Autodesk Inventor part; units mm, degrees
ref_plane "YZ Plane" through (0, 0, 0) normal (1, 0, 0) x (0, 1, 0)
ref_plane "XZ Plane" through (0, 0, 0) normal (0, 1, 0) x (-1, 0, 0)
ref_plane "XY Plane" through (0, 0, 0) normal (0, 0, 1) x (1, 0, 0)
sketch "Sketch1" plane through (0, 0, 0) normal (0, 1, 0) x (-1, 0, 0)
  circle A0 centre (0, 0) radius 9.525
  dimension "d0" = 19.05
extrude "Extrusion1" add sketch "Sketch1" along normal mid plane 30.48
sketch "Sketch3" plane through (0, 15.24, 0) normal (0, 1, 0) x (1, 0, 0)
  point P0 (0, 0)
  point P1 (0, 0)
hole "Hole1" at (0, 15.24, 0) direction (0, -1, 0) diameter 7.9375 end through all
sketch "Sketch4" plane through (0, 15.24, 0) normal (0, 1, 0) x (1, 0, 0)
  point P0 (0, 0)
  point P1 (0, 0)
hole "Hole2" at (0, 15.24, 0) direction (0, -1, 0) diameter 12.3031 depth 10.16 tip angle 118
sketch "Sketch5" plane through (0, 15.24, 0) normal (0, 1, 0) x (1, 0, 0)
  circle A0 centre (0, 0) radius 6.3627
  dimension "d20" = 12.7254
extrude "Extrusion3" cut sketch "Sketch5" against normal blind 11.43
sketch "Sketch6" plane through (0, 15.24, 0) normal (0, 1, 0) x (1, 0, 0)
  circle A0 centre (0, 0) radius 6.477
  dimension "d23" = 12.954
extrude "Extrusion4" cut sketch "Sketch6" against normal blind 2.54
sketch "Sketch7" plane through (0, -15.24, 0) normal (0, -1, 0) x (1, 0, 0)
  circle A0 centre (0, 0) radius 9.525
  circle A1 centre (0, 0) radius 9.525
  circle A2 centre (0, 0) radius 5.5753
  dimension "d26" = 11.1506
extrude "Extrusion5" cut sketch "Sketch7" against normal blind 15.24
sketch "Sketch9" plane through (0, 0, 0) normal (0, 0, 1) x (1, 0, 0)
  line L0 (3.9688, -15.24) -> (-3.9688, -15.24)
  line L1 (0, -15.24) -> (0, -4.064) construction
  line L2 (0, -15.24) -> (11.176, -15.24) construction
  line L3 (0, -4.064) -> (5.5753, -4.064) construction
  line L4 (5.5753, -15.24) -> (5.5753, 0)
  line L5 (5.7023, -2.794) -> (5.4483, -2.794)
  line L6 (5.4483, -2.794) -> (5.4483, -5.334)
  line L7 (5.4483, -5.334) -> (5.7023, -5.334)
  line L8 (5.7023, -5.334) -> (5.7023, -2.794)
  line L9 (5.7023, -2.794) -> (5.4483, -5.334) construction
  line L10 (5.4483, -2.794) -> (5.7023, -5.334) construction
  point P0 (0, 0)
  dimension "d35" = 11.176
  dimension "d36" = 90
  dimension "d38" = 90
  dimension "d39" = 0.254
  dimension "d40" = 2.54
revolve "Revolution1" cut sketch "Sketch9" angle 360 about axis through (0, -15.24, 0) along (0, 1, 0)
chamfer "Chamfer2" distance 1.5875 angle 45 1 edges at (9.525, 0, 0)
properties part number "fridge bushing" material "Brass"
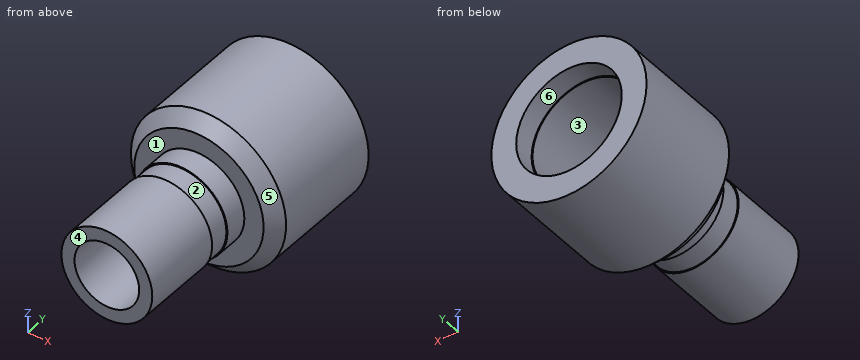
Geometry: final body of the model. Coordinates: model frame, mm. Face numbers are marked on the shaded views. A direction names the side the tool comes from. Coordinates: 2 decimals unless noted, no trailing zeros. Order: outer loops, then holes, each group sorted by start corner. A loop starts at its lowest first (then second) coordinate and runs counter-clockwise, first axis right, second up.
1) Section C-C (y = 13.5). Return loops of the section in (x, z) (3 decimals).
Result sheet:
outline: circle Ø19.05 at (0, 0); hole circle Ø12.954 at (0, 0)
2) First-contact query: P1, Ø5.5, axis at x = -2, z = 0, coming from the +Y side; P2, Ø1, axis at y = -11, z = 3.5, coming from the -X side; P3, Ø2, axis at y = -0.5, z = -0.5, coming from the +X side; P4, Ø3, axis at y = 2.5, z = -1, coming from the +X side (3 decimals). Flat tips, straight axial feed; report the tip coordinate or a pass-through.
Result sheet:
P1: stops at y = 3.81
P2: stops at x = -4.7
P3: stops at x = 8.42
P4: stops at x = 9.525
3) Draft query along Z for the marked faces 4, 5 and 6. Return one class per face: released by +Z, released by -Z, zero draft, split by the parting line, or undercut.
Result sheet:
face 4: zero draft
face 5: split by the parting line
face 6: undercut
4) Ray query, probe 1 along Z at (x, y) = (0, 14.25) (3 decimals); probe 2 along Z at (x, y) = (0, 7.75) (3 decimals); probe 3 along X at (y, z) = (-5, 0). Return the intervals inside material, ascending.
Result sheet:
probe 1: z = -9.525 to -6.477, 6.477 to 9.525
probe 2: z = -9.525 to -6.363, 6.363 to 9.525
probe 3: x = -5.45 to -3.97, 3.97 to 5.45
5) Section D-D (y = 6). Return loops of the section in (x, z) (3 decimals).
Result sheet:
outline: circle Ø19.05 at (0, 0); hole circle Ø12.725 at (0, 0)
6) Set-up query: the marked faces 1, 2 and 3. Return all of +Z, -Z, +X, -X, +Y, -Y with unobstructed straight access to the full face (end or side cutting, diameter ignored); none if empty.
Result sheet:
face 1: -Y
face 2: none
face 3: +Y
